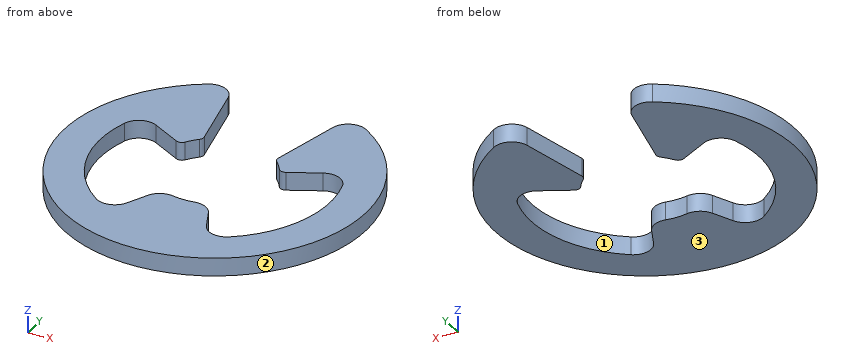
Autodesk Inventor part; units mm, degrees
ref_plane "YZ Plane" through (0, 0, 0) normal (1, 0, 0) x (0, 1, 0)
ref_plane "XZ Plane" through (0, 0, 0) normal (0, 1, 0) x (-1, 0, 0)
ref_plane "XY Plane" through (0, 0, 0) normal (0, 0, 1) x (1, 0, 0)
sketch "Sketch1" plane through (0, 0, 0) normal (0, 0, 1) x (1, 0, 0)
  circle A0 centre (0, 0) radius 1.1906
  circle A1 centre (0, 0) radius 3.175
  dimension "d0" = 2.3813
  dimension "d1" = 6.35
extrude "Extrusion1" add sketch "Sketch1" along normal mid plane 0.381
sketch "Sketch2" plane through (0, 0, 0.1905) normal (0, 0, 1) x (1, 0, 0)
  circle A0 centre (0, 0) radius 1.1906 construction
  circle A1 centre (0, 0) radius 3.175
  line L0 (0, -4.445) -> (0, 4.445)
  line L1 (-4.445, 0) -> (4.445, 0)
  circle A2 centre (0, 0) radius 1.1906 construction
  line L2 (-0.635, 0.3107) -> (0.635, 0.3107)
  line L3 (0.635, 0.3107) -> (1.27, 3.175)
  line L4 (1.27, 3.175) -> (-1.27, 3.175)
  line L5 (-1.27, 3.175) -> (-0.635, 0.3107)
  circle A3 centre (0, 0) radius 3.175
  dimension "d4" = 1.27
  dimension "d5" = 2.54
  dimension "d6" = 25
extrude "Extrusion2" cut sketch "Sketch2" against normal through all contours L3 L2 L0 A1 | A1 L4 L3 | L0 L2 L5 A1 | A1 L5 L4
sketch "Sketch3" plane through (0, 0, 0.1905) normal (0, 0, 1) x (1, 0, 0)
  arc A0 (-1.2163, 2.9328) -> (1.2163, 2.9328) centre (0, 0) ccw
  arc A1 (-2.1409, 1.1132) -> (2.1409, 1.1132) centre (0, 0) ccw
  line L0 (-4.445, 0) -> (4.445, 0)
  line L1 (0, -4.3966) -> (0, 4.1543)
  line L2 (-2.1409, 1.1132) -> (-1.0566, 0.5487)
  arc A2 (-0.7678, 0.9099) -> (0.7678, 0.9099) centre (0, 0) ccw
  line L3 (2.1409, 1.1132) -> (1.0566, 0.5487)
  line L4 (-0.7678, 0.9099) -> (-1.2163, 2.9328)
  line L5 (-0.5029, -1.0792) -> (-1.0195, -2.187)
  line L6 (0.5029, -1.0792) -> (1.0195, -2.187)
  dimension "d9" = 0.762
  dimension "d10" = 50
  dimension "d11" = 50
  dimension "d12" = 2.1133
  dimension "d13" = 1.0058
extrude "Extrusion3" cut sketch "Sketch3" against normal through all contours L0 A2 L5 A1 | A1 L2 A2 L0 | L0 A2 L3 A1 | A1 L6 A2 L0
fillet "Fillet1" radius 0.381 8 edges at (-1.2163, 2.9328, 0) (1.2163, 2.9328, 0) (-2.1409, 1.1132, 0) (2.1409, 1.1132, 0) (-1.0195, -2.187, 0) (1.0195, -2.187, 0) (0.5029, -1.0792, 0) (-0.5029, -1.0792, 0)
fillet "Fillet2" radius 0.127 4 edges at (-0.7678, 0.9099, 0) (-1.0566, 0.5487, 0) (0.7678, 0.9099, 0) (1.0566, 0.5487, 0)
properties part number "E-Clip"
Geometry: final body of the model. Coordinates: model frame, mm. Face numbers are marked on the shaded views. Round coordinates to 2 decimals unless told otherwise and drop trailing zeros. Order: outer loops, then holes, each group sorted by start corner. A loop starts at its lowest first (then second) coordinate and runs counter-clockwise, first axis right, second up.
Q1. Section B-B, the plane z = 0. Output: boundary loops of the cut face in (x, y) (3 decimals), and give its area (3 significant figures).
Result sheet:
outline: (-2.312, 0.692) arc R0.381 cw to (-1.771, 0.921) - (-1.164, 0.605) arc R0.127 ccw to (-0.999, 0.648) arc R1.191 cw to (-0.82, 0.863) arc R0.127 ccw to (-0.784, 0.982) - (-1.11, 2.451) arc R0.381 ccw to (-1.684, 2.692) arc R3.175 ccw (long way) to (1.684, 2.692) arc R0.381 ccw to (1.11, 2.451) - (0.784, 0.982) arc R0.127 ccw to (0.82, 0.863) arc R1.191 cw to (0.999, 0.648) arc R0.127 ccw to (1.164, 0.605) - (1.771, 0.921) arc R0.381 cw to (2.312, 0.692) arc R2.413 cw to (1.411, -1.957) arc R0.381 cw to (0.843, -1.809) - (0.644, -1.382) arc R0.381 ccw to (0.226, -1.169) arc R1.191 cw to (-0.226, -1.169) arc R0.381 ccw to (-0.644, -1.382) - (-0.843, -1.809) arc R0.381 cw to (-1.411, -1.957) arc R2.413 cw to start
area: 16.0 mm2
Q2. Mould query, pull axis Y, two halves, no side actions, for the marked faces 1, 2 and 3. Classes: released by +Y, released by -Y, zero draft, split by the parting line, or undercut.
Result sheet:
face 1: undercut
face 2: split by the parting line
face 3: zero draft
Q3. Material intervals for probe 1 along X at (y, z) = (-1.8, 0.15); probe 2 along X at (y, z) = (-1.95, 0); probe 3 along Y at (x, z) = (0, 0) (3 decimals), sorted ascending.
Result sheet:
probe 1: x = -2.62 to -1.61, -0.84 to 0.84, 1.61 to 2.62
probe 2: x = -2.51 to -1.42, -0.96 to 0.96, 1.42 to 2.51
probe 3: y = -3.175 to -1.191
Q4. Section C-C, the plane y = 1.15. Output: boundary loops of the cut face in (x, z).
Result sheet:
outline: (-2.96, -0.19) - (-0.82, -0.19) - (-0.82, 0.19) - (-2.96, 0.19) - close; (0.82, -0.19) - (2.96, -0.19) - (2.96, 0.19) - (0.82, 0.19) - close
